Geometry: see drawing. Coordinates: mm, zero at the bounding-box minimum. Coordinates: 2 decimals unless noted, no trailing zeros. Write each loop counter-clockwise with the first axis right and the second up, starting at its lowest first coordinate (ties: lowest second). Pieces come first, ordered by that corner, then holes.
1) Section query C-C (y = 6.75). Output: boundary loops of the cut face in (x, z).
2) Section query A-A (x = 6.75). Output: boundary loops of the cut face in (y, z), then the cut area to 3 significant figures.
3) Draft query along X for the marked faces 1, 2 and 3. Return one class per face: pulls with the +X half, pulls with the -X half, needs draft (parallel to the pull), parting line crosses it, or undercut.
4) Section query B-B (z = 6.75). Output: boundary loops of the cut face in (x, y).
5) Pin query (flat end, axial travel): pin 1 Ø6 at (x, z) = (2, 4.5) entering from -Y; pin 2 Ø6 at (x, y) = (5.5, 6) entering from +Z; pin 3 Ø4 at (x, z) = (9, 4.5) entering from -Y; pin 4 Ø4 at (y, z) = (6, 8.5) entering from +X. Return the tip coordinate at first contact, or that it passes through.
6) Line query: L1, parallel to X at y = 7.75, z = 6.75; L2, parallel to Z at x = 8, y = 6.25; L3, parallel to X at y = 8.25, z = 8.5. Output: solid intervals per line, ascending.
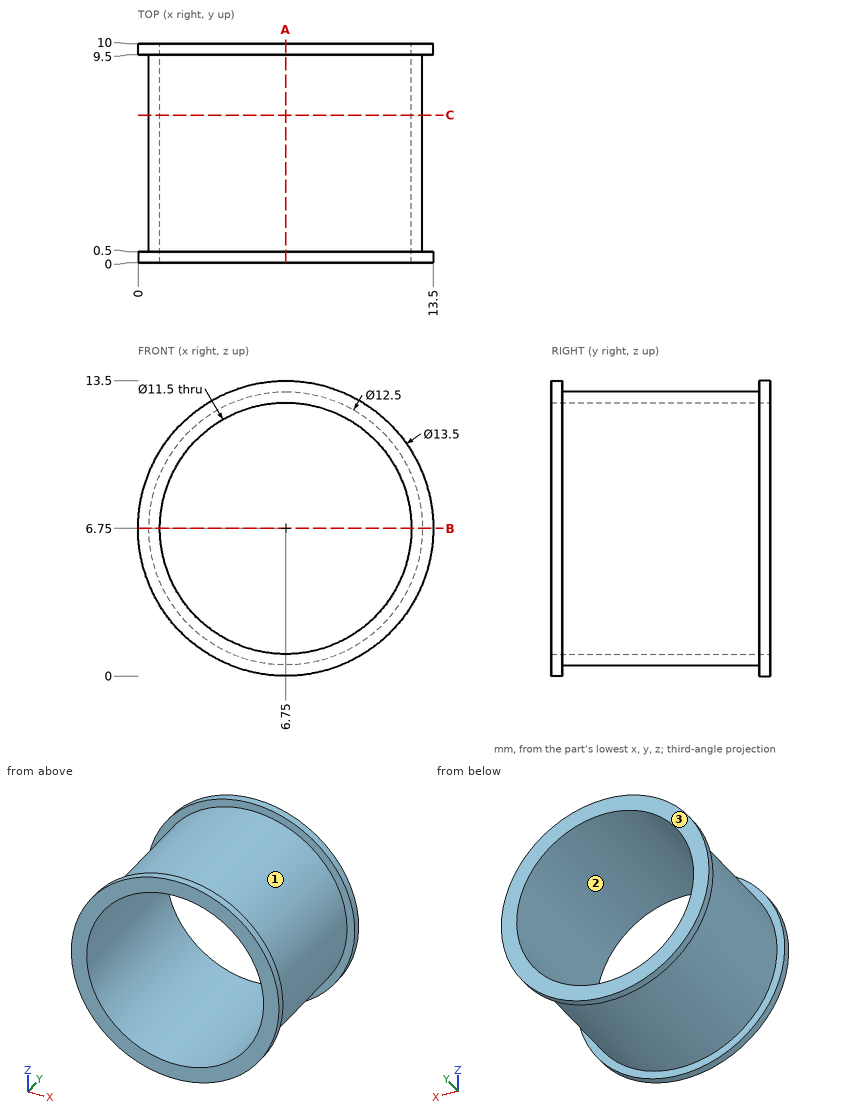
Answer:
1. outline: circle Ø12.5 at (6.75, 6.75); hole circle Ø11.5 at (6.75, 6.75)
2. outline: (0, 0) - (0.5, 0) - (0.5, 0.5) - (9.5, 0.5) - (9.5, 0) - (10, 0) - (10, 1) - (0, 1) - close; (0, 12.5) - (10, 12.5) - (10, 13.5) - (9.5, 13.5) - (9.5, 13) - (0.5, 13) - (0.5, 13.5) - (0, 13.5) - close
2. area: 11.0 mm2
3. face 1: parting line crosses it
3. face 2: undercut
3. face 3: needs draft
4. outline: (0, 0) - (1, 0) - (1, 10) - (0, 10) - (0, 9.5) - (0.5, 9.5) - (0.5, 0.5) - (0, 0.5) - close; (12.5, 0) - (13.5, 0) - (13.5, 0.5) - (13, 0.5) - (13, 9.5) - (13.5, 9.5) - (13.5, 10) - (12.5, 10) - close
5. pin 1: stops at y = 0
5. pin 2: stops at z = 13
5. pin 3: passes through
5. pin 4: stops at x = 13
6. L1: x = 0.5 to 1, 12.5 to 13
6. L2: z = 0.63 to 1.14, 12.36 to 12.87
6. L3: x = 0.75 to 1.27, 12.23 to 12.75
